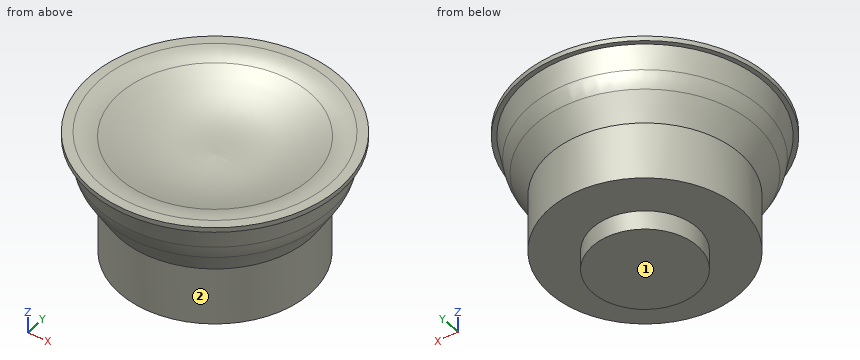
from build123d import *

# Parameters (mm, degrees)
F0_R     = 11
F1_DEPTH = 4
F2_R     = 20
F2_R_2   = 11
F3_DEPTH = 12


with BuildPart() as f1:
    # F0 (on Top) → F1 (new body)
    with BuildSketch(Plane.XY):
        Circle(F0_R)
    extrude(amount=F1_DEPTH)

    # F2 (on face) → F3 (join)
    with BuildSketch(Plane.XY.offset(4)):
        Circle(F2_R)
        Circle(F2_R_2, mode=Mode.SUBTRACT)
        Circle(F2_R_2)
    extrude(amount=F3_DEPTH)

    # F4 (on Front) → F5 (revolve)
    with BuildSketch(Plane.XZ):
        with BuildLine():
            Line((26.2435501542, 30), (24.2435501542, 30))
            ThreePointArc((24.2435501542, 30), (22.1053432538, 29.7687292547), (20.066037294, 29.0856142502))
            add(Edge.make_bspline(
                [(0, 25.1485239714), (3.3020219353, 24.9547299716), (9.7317137995, 24.5773746031), (16.670969278, 27.5245816212), (20.066037294, 29.0856142502)],
                knots=[0, 0, 0, 0, 0.4694356931, 0.9140844354, 0.9140844354, 0.9140844354, 0.9140844354], degree=3))
            Line((0, 25.1485239714), (0, 16))
            Line((0, 16), (20, 16))
            Line((20, 16), (23.0461187635, 20.9651674984))
            ThreePointArc((23.0461187635, 20.9651674984), (23.82328384, 22.5212025281), (24.3190746637, 24.1883623971))
            Line((24.3190746637, 24.1883623971), (25.3043714911, 29))
            Line((25.3043714911, 29), (26.2435501542, 29))
            Line((26.2435501542, 29), (26.2435501542, 30))
        make_face()
    revolve(axis=Axis((0, 0, 21.7276830226), (0, 0, 1)))


solid = f1.part
Geometry check sheet. Reference: the model listing, model coordinates, mm. Face numbers are marked on the shaded views. A direction names the side the tool comes from. Round coordinates to 2 decimals unless told otherwise and drop trailing zeros. Loops run counter-clockwise (first coordinate to the right, second up) from the corner with the lowest first, then second, coordinate; pieces in that order, holes last.
Item 1: Access from +Z, -Z, +X, -X, +Y, -Y to the whole of each face (thin tool, end or side, straight path). Record for the marked faces 1 and 2.
Item 2: Thickness scan on line 1 (Y direction, x = 0, z = 8); line 2 (Z direction, x = 1, y = -4.5); line 3 (X direction, y = -6.5, z = 21.5). Record the ranges inside material, lowest first.
Item 3: Gauge pin test, flat ends, axial feed: pin 1 (8 mm diameter, centred on x = 19.5, y = -16.5, fed in from -Z); pin 2 (8 mm diameter, centred on x = -5, z = 9.5, fed in from +Y) (3 decimals); pin 3 (3 mm diameter, centred on y = -4, z = 4, fed in from +X). Record the tip position at first contact, or that the pin passes through.
Item 4: Cross-section at A-A on z = 9.5. Record the boundary of the cut face in (x, y), then the cut area to 3 significant figures.
Answer sheet:
1. face 1: -Z, +X, -X, +Y, -Y
1. face 2: -Z
2. line 1: y = -20 to 20
2. line 2: z = 0 to 24.97
2. line 3: x = -22.43 to 22.43
3. pin 1: stops at z = 18.52
3. pin 2: stops at y = 19.975
3. pin 3: stops at x = 19.84
4. outline: circle Ø40 at (0, 0)
4. area: 1,260 mm2
